Autodesk Inventor part; units mm, degrees
ref_plane "YZ Plane" through (0, 0, 0) normal (1, 0, 0) x (0, 1, 0)
ref_plane "XZ Plane" through (0, 0, 0) normal (0, 1, 0) x (-1, 0, 0)
ref_plane "XY Plane" through (0, 0, 0) normal (0, 0, 1) x (1, 0, 0)
sketch "Sketch1" plane through (0, 0, 0) normal (0, 1, 0) x (-1, 0, 0)
  line L0 (0, 0) -> (-25.4, 0)
  line L1 (-25.4, 0) -> (-25.4, -25.4)
  line L2 (-25.4, -25.4) -> (0, -25.4)
  line L3 (0, -25.4) -> (0, 0)
  line L4 (0, 0) -> (0, -6.35)
  line L5 (0, -6.35) -> (-6.35, -6.35)
  line L6 (-6.35, -6.35) -> (-6.35, -19.05)
  line L7 (0, -12.7) -> (-12.446, -12.7)
  circle A0 centre (-6.35, -6.35) radius 2.25
  circle A1 centre (-6.35, -19.05) radius 2.25
  circle A2 centre (-12.7, -12.7) radius 2.25
  circle A3 centre (-12.446, -12.7) radius 2.25
  dimension "d0" = 25.4
  dimension "d1" = 25.4
  dimension "d2" = 6.35
  dimension "d3" = 6.35
  dimension "d4" = 12.7
  dimension "d5" = 12.446
  dimension "d6" = 4.5
  dimension "d7" = 4.5
  dimension "d8" = 4.5
  dimension "d20" = 4.5
extrude "Extrusion1" add sketch "Sketch1" along normal blind 6.35 contours L3 L5 A0 L6 L7 L2 L1 L0 | L3 L7 L6 A0 L5 | A3 A2 picked at (-14.7705, -12.7)
sketch "Sketch2" plane through (0, 6.35, 0) normal (0, 1, 0) x (1, 0, 0)
  circle A0 centre (12.7, 12.7) radius 2.25
  line L0 (0, 25.4) -> (0, 0)
  line L1 (0, 0) -> (25.4, 0)
  line L2 (25.4, 0) -> (25.4, 25.4)
  line L3 (25.4, 25.4) -> (0, 25.4)
  line L4 (0, 25.4) -> (0, 0)
  circle A1 centre (6.35, 19.05) radius 2.25
  circle A2 centre (6.35, 6.35) radius 2.25
  line L5 (12.7, 12.7) -> (-15.325, 12.7)
  circle A3 centre (-15.325, 12.7) radius 2.25
  line L6 (0, 19.05) -> (-20.32, 19.05)
  line L7 (-20.32, 19.05) -> (-20.32, 6.35)
  line L8 (-20.32, 6.35) -> (0, 6.35)
  line L9 (0, 6.35) -> (0, 19.05)
  point P0 (0, 6.35)
  dimension "d11" = 28.025
  dimension "d12" = 4.5
  dimension "d13" = 20.32
extrude "Extrusion2" add sketch "Sketch2" against normal blind 6.35 contours L0 L8 L7 L6
sketch "Sketch3" plane through (0, 6.35, 0) normal (0, 1, 0) x (1, 0, 0)
  circle A0 centre (12.7, 12.7) radius 2.25
  circle A1 centre (6.35, 19.05) radius 2.25
  circle A2 centre (6.35, 6.35) radius 2.25
  circle A3 centre (6.35, 19.05) radius 3.81
  circle A4 centre (6.35, 6.35) radius 3.81
  point P0 (0, 0)
  dimension "d16" = 7.62
  dimension "d17" = 7.62
extrude "Extrusion3" cut sketch "Sketch3" against normal blind 5.08 contours A1 | A2 | A3 | A4
properties part number "DovetailSampleHolderToKB1X1TMagneticHolder"
Check sheet for the modelled part. Datum: model origin and axes. Units: mm. A direction names the side the tool comes from. Round coordinates to 2 decimals unless told otherwise and drop trailing zeros. Loops run counter-clockwise (first coordinate to the right, second up) from the corner with the lowest first, then second, coordinate; pieces in that order, holes last. Notation, with made-up numbers: M 12.25,54 L 69.25,54 A20 ccw 69.25,90 Z; hole C 11.25,61 d10. An arc over 180 degrees is marked long. One line per item, written item: value.
(1) Release check for a two-part mould opening along Z. For faces 6 (the face through (5.854, 3.846, -10.128)), 7 (the face through (-10, 3, -19.05)), 8 (the face through (-10, 3, -6.35)) record: +Z half, -Z half, draft (parallel to the pull), parting line (faces both ways), or undercut.
Computed values:
face 6: undercut
face 7: -Z half
face 8: +Z half
(2) Sectioned sample at A-A, the plane x = 6.35. Record the cut outline in (y, z), then the cut area to 3 significant figures.
Computed values:
outline: M 0,-25.4 L 6.35,-25.4 L 6.35,-22.86 L 1.27,-22.86 L 1.27,-21.3 L 0,-21.3 Z; M 0,-16.8 L 1.27,-16.8 L 1.27,-15.24 L 6.35,-15.24 L 6.35,-10.16 L 1.27,-10.16 L 1.27,-8.6 L 0,-8.6 Z; M 0,-4.1 L 1.27,-4.1 L 1.27,-2.54 L 6.35,-2.54 L 6.35,0 L 0,0 Z
area: 72.4 mm^2
(3) Sectioned sample at C-C, the plane y = 3. Record the cut outline in (x, z) (3 decimals), then the cut area to 3 significant figures.
Computed values:
outline: M -20.32,-19.05 L 0,-19.05 L 0,-25.4 L 25.4,-25.4 L 25.4,0 L 0,0 L 0,-6.35 L -20.32,-6.35 Z; hole C -15.325,-12.7 d4.5; hole C 6.35,-19.05 d7.62; hole C 6.35,-6.35 d7.62; hole C 12.446,-12.7 d4.5
area: 780 mm^2
(4) Sectioned sample at D-D, the plane z = -5.5. Record the cut outline in (x, y), then the cut area to 3 significant figures.
Computed values:
outline: M 0,0 L 4.27,0 L 4.27,1.27 L 2.64,1.27 L 2.64,6.35 L 0,6.35 Z; M 8.43,0 L 25.4,0 L 25.4,6.35 L 10.06,6.35 L 10.06,1.27 L 8.43,1.27 Z
area: 118 mm^2
(5) Access from +Z, -Z, +X, -X, +Y, -Y to the whole of each face (thin tool, end or side, straight path). Record for faces 1 (the face through (7, 6.35, -13)), 2 (the face through (0, 3, -3)), 3 (the face through (5.854, 3.846, -22.828)), 4 (the face through (25.4, 3, -13)), 5 (the face through (0, 3, -22)).
Computed values:
face 1: +Z, -Z, +X, -X, +Y
face 2: +Z, -X, +Y, -Y
face 3: +Y
face 4: +Z, -Z, +X, +Y, -Y
face 5: -Z, -X, +Y, -Y
(6) Sectioned sample at B-B, the plane z = -12.7. Record the cut outline in (x, y) (3 decimals), then the cut area to 3 significant figures.
Computed values:
outline: M -20.32,0 L -17.575,0 L -17.575,6.35 L -20.32,6.35 Z; M -13.075,0 L 10.196,0 L 10.196,6.35 L -13.075,6.35 Z; M 14.696,0 L 25.4,0 L 25.4,6.35 L 14.696,6.35 Z
area: 233 mm^2
(7) Thickness scan on line 1 (Z direction, x = 6.35, y = 0.5); line 2 (X direction, y = 1.5, z = -6.25); line 3 (Z direction, x = 5, y = 1.75). Record the ranges inside material, lowest first.
Computed values:
line 1: z = -25.4 to -21.3, -16.8 to -8.6, -4.1 to 0
line 2: x = 0 to 2.54, 10.16 to 25.4
line 3: z = -25.4 to -22.61, -15.49 to -9.91, -2.79 to 0
(8) Depth check by flat-ended pin: pin 1 Ø3 at (y, z) = (3.5, -21.5) entering from -X. Enter the tip coordinate at first touch or a pass-through.
Computed values:
pin 1: stops at x = 0
